Here's the drawing with two shaded views (mm, measured from the low corner). I have some questions. A direction names the side the tool comes from. Give positions to 0.01 mm unless a question says otherwise; leave off trailing zeros. Order: outer loops, then holes, each group sorted by start corner. A loop starts at its lowest first (then second) coordinate and runs counter-clockwise, first axis right, second up. Notation, with made-up numbers: M -23,80 L -13,80 A35 cw -13,116 Z; hole C 74.25,12 d2. An arc over 180 degrees is marked long. Use a Markdown table: item, result. Add a question column.
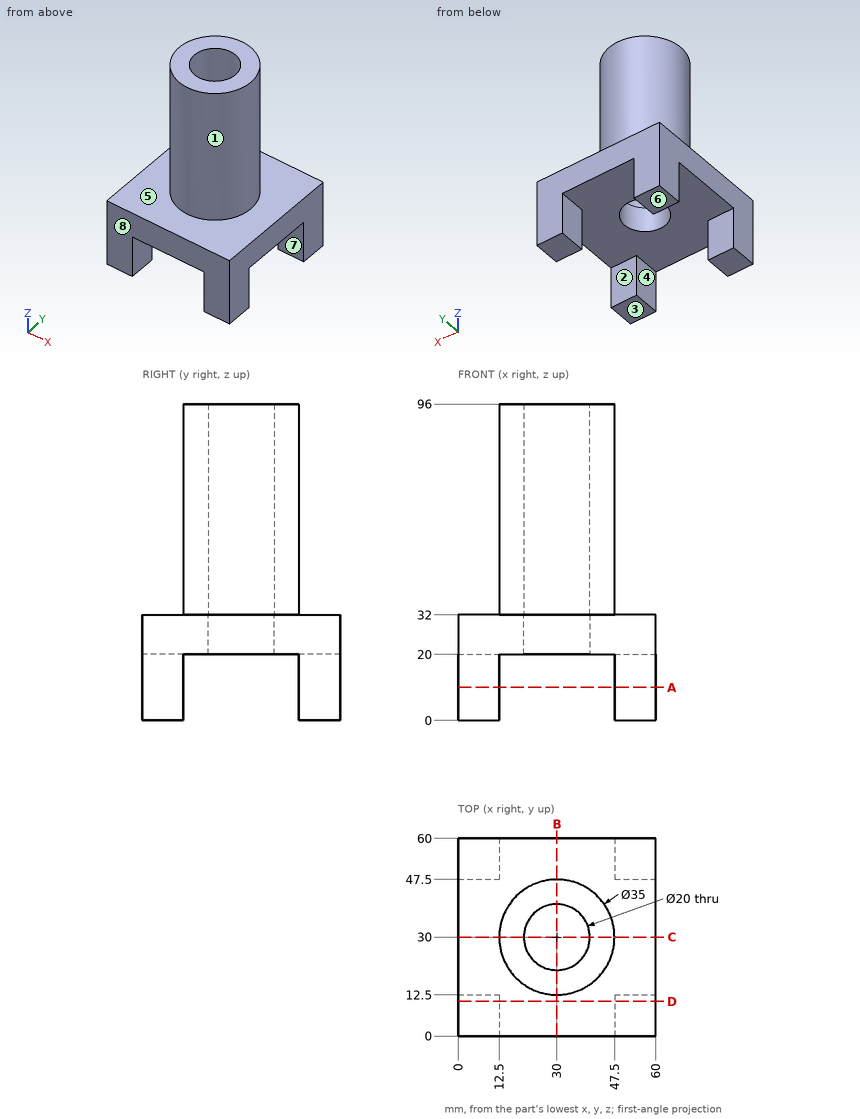
1) For pin 1 (5 mm diameter, centred on y = 20.5, z = 84.5, fed in from -X); pin 2 (10 mm diameter, centred on y = 41.5, z = 77.5, fed in from +X); pin 3 (1 mm diameter, centred on y = 42, z = 57, fed in from -X), each with a flat end and sliding along its axis, tell me the tip position at first contact or that it passes through.
2) Suppose I cut it at A-A on z = 10. Please give me the cut outline in (x, y).
3) We'd pull the mould along Y, two halves only. Please class the marked faces 1, 2 and 3: pulls with the +Y half, pulls with the -Y half, needs draft (parallel to the pull), parting line crosses it, or undercut.
4) Please list where these lines run through material, in increasing order: line 1 (Y direction, x = 30, z = 24); line 2 (X direction, y = 55, z = 18); line 3 (X direction, y = 29.5, z = 70). Write a range as from..to.
5) For the marked faces 4, 5, 6, 7 and 8, which set-ups out of +Z, -Z, +X, -X, +Y, -Y let a thin tool reach every point of the face, with its end or its side?
6) Suppose I cut it at D-D on y = 10.5. Please give me the cut outline in (x, z).
7) Suppose I cut it at B-B on x = 30. Please give me the cut outline in (y, z).
Values found:
| question | item | result |
|---|---|---|
| 1 | pin 1 | stops at x = 13.96 |
| 1 | pin 2 | stops at x = 46.25 |
| 1 | pin 3 | stops at x = 16.81 |
| 2 | outline | M 0,0 L 12.5,0 L 12.5,12.5 L 0,12.5 Z; M 0,47.5 L 12.5,47.5 L 12.5,60 L 0,60 Z; M 47.5,0 L 60,0 L 60,12.5 L 47.5,12.5 Z; M 47.5,47.5 L 60,47.5 L 60,60 L 47.5,60 Z |
| 3 | face 1 | parting line crosses it |
| 3 | face 2 | undercut |
| 3 | face 3 | needs draft |
| 4 | line 1 | y = 0..20, 40..60 |
| 4 | line 2 | x = 0..12.5, 47.5..60 |
| 4 | line 3 | x = 12.51..20.01, 39.99..47.49 |
| 5 | face 4 | -Z, +Y, -Y |
| 5 | face 5 | +Z |
| 5 | face 6 | -Z, +X, -X, +Y, -Y |
| 5 | face 7 | -Z, +X, -X |
| 5 | face 8 | +Z, -Z, +X, -X, -Y |
| 6 | outline | M 0,0 L 12.5,0 L 12.5,20 L 47.5,20 L 47.5,0 L 60,0 L 60,32 L 0,32 Z |
| 7 | outline | M 0,20 L 20,20 L 20,96 L 12.5,96 L 12.5,32 L 0,32 Z; M 40,20 L 60,20 L 60,32 L 47.5,32 L 47.5,96 L 40,96 Z |
